from build123d import *

# Parameters (mm, degrees)
SKETCH1_R                = 1.75
SKETCH1_W                = 7.2
SKETCH1_H                = 5.4
BOSS_EXTRUDE1_DEPTH      = 5
FILLET5_RADIUS           = 10
FILLET5_LENGTH           = 5
FILLET2_R                = 5.4
FILLET6_R                = 5.4
SKETCH3_W                = 35
SKETCH3_H                = 20
SKETCH3_W_2              = 23
SKETCH3_H_2              = 13
BOSS_EXTRUDE4_DEPTH      = 5
SKETCH5_W                = 23
SKETCH5_H                = 13
CUT_EXTRUDE1_DEPTH       = 2.74
CUT_EXTRUDE2_DEPTH       = 76.166481892
FILLET9_R                = 4
BOSS_EXTRUDE7_DEPTH      = 26
BOSS_EXTRUDE7_DEPTH_BACK = 5
SKETCH7_W                = 5
SKETCH7_H                = 20
SKETCH8_R                = 2.75
CUT_EXTRUDE3_DEPTH       = 79.677569866
FILLET10_R               = 10
SKETCH9_R                = 1
CUT_EXTRUDE4_DEPTH       = 7
BOSS_EXTRUDE8_DEPTH      = 5
SKETCH11_R               = 1.3
CUT_EXTRUDE5_DEPTH       = 5
SKETCH12_W               = 14
SKETCH12_H               = 7
CUT_EXTRUDE6_DEPTH       = 4
FILLET11_R               = 3.5


with BuildPart() as part:
    # Sketch1 → Boss-Extrude1 (new body)
    # profile 1 of 4: a face of its own
    with BuildSketch(Plane(origin=(0, 0, 0), x_dir=(1, 0, 0), z_dir=(0, 1, 0))):
        with BuildLine():
            Line((3.05, 25), (0, 25))
            Line((0, 25), (0, 15))
            Line((0, 15), (10, 0))
            Line((10, 0), (26, 0))
            Line((26, 0), (36, 15))
            Line((36, 15), (60, 15))
            Line((60, 15), (60, 25))
            Line((60, 25), (44.5, 25))
            Line((44.5, 25), (44.5, 19.6))
            Line((44.5, 19.6), (37.3, 19.6))
            Line((37.3, 19.6), (26.5, 19.6))
            Line((26.5, 19.6), (26.5, 25))
            Line((26.5, 25), (6.55, 25))
            ThreePointArc((6.55, 25), (4.8, 23.25), (3.05, 25))
        make_face()
        with Locations(Location((13, 5, 0), (0, 0, 270))):
            Circle(SKETCH1_R, mode=Mode.SUBTRACT)
        with Locations(Location((23, 5, 0), (0, 0, 270))):
            Circle(SKETCH1_R, mode=Mode.SUBTRACT)
    # profile 2 of 4: a face of its own
    with BuildSketch(Plane(origin=(0, 0, 0), x_dir=(1, 0, 0), z_dir=(0, 1, 0))):
        with BuildLine():
            Line((10, 45), (0, 33.819660113))
            Line((0, 33.819660113), (0, 25))
            Line((0, 25), (3.05, 25))
            ThreePointArc((3.05, 25), (4.8, 26.75), (6.55, 25))
            Line((6.55, 25), (26.5, 25))
            Line((26.5, 25), (26.5, 30.4))
            Line((26.5, 30.4), (37.3, 30.4))
            Line((37.3, 30.4), (44.5, 30.4))
            Line((44.5, 30.4), (44.5, 25))
            Line((44.5, 25), (60, 25))
            Line((60, 25), (60, 35))
            Line((60, 35), (36, 35))
            Line((36, 35), (26, 45))
            Line((26, 45), (10, 45))
        make_face()
    # profile 3 of 4: a face of its own
    with BuildSketch(Plane(origin=(0, 0, 0), x_dir=(1, 0, 0), z_dir=(0, 1, 0))):
        with Locations((40.9, 27.7)):
            Rectangle(SKETCH1_W, SKETCH1_H)
    # profile 4 of 4: a face of its own
    with BuildSketch(Plane(origin=(0, 0, 0), x_dir=(1, 0, 0), z_dir=(0, 1, 0))):
        with Locations((40.9, 22.3)):
            Rectangle(SKETCH1_W, SKETCH1_H)
    extrude(amount=BOSS_EXTRUDE1_DEPTH)

    # Fillet5: full round fillet: the end face becomes a half cylinder, R = half its width
    fillet5_face = Plane((60, 2.5, -25), x_dir=(0, -1, 0), z_dir=(1, 0, 0))  # on the end face: x along it, z out of the body
    fillet5_slab = fillet5_face.offset(-FILLET5_RADIUS / 2) * Box(FILLET5_LENGTH, 2 * FILLET5_RADIUS, FILLET5_RADIUS, mode=Mode.PRIVATE)  # the body's end, R deep
    fillet5_round = Plane((50, 2.5, -25), x_dir=(1, 0, 0), z_dir=(0, -1, 0)) * Cylinder(FILLET5_RADIUS, FILLET5_LENGTH, mode=Mode.PRIVATE)  # its axis R under the face
    add(fillet5_slab - fillet5_round, mode=Mode.SUBTRACT)

    # Fillet2
    fillet2_edges = [part.edges().sort_by_distance(p)[0] for p in [
        (26.5, 2.5, -30.4),
        (26.5, 2.5, -19.6),
    ]]
    fillet(fillet2_edges, radius=FILLET2_R - 0.0001)  # a hair under: the kernel refuses the full size

    # Fillet6
    fillet6_edges = [part.edges().sort_by_distance(p)[0] for p in [
        (37.3, 2.5, -19.6),
        (37.3, 2.5, -30.4),
    ]]
    fillet(fillet6_edges, radius=FILLET6_R - 0.0001)  # a hair under: the kernel refuses the full size

    # Sketch3 → Boss-Extrude4 (add)
    with BuildSketch(Plane.XZ):
        with Locations((26.9, -25)):
            Rectangle(SKETCH3_W, SKETCH3_H)
        with Locations((26.9, -25)):
            Rectangle(SKETCH3_W_2, SKETCH3_H_2, mode=Mode.SUBTRACT)
    extrude(amount=BOSS_EXTRUDE4_DEPTH)

    # Sketch5 → Cut-Extrude1 (cut)
    with BuildSketch(Plane.XZ):
        with Locations((26.9, -25)):
            Rectangle(SKETCH5_W, SKETCH5_H)
    extrude(amount=-CUT_EXTRUDE1_DEPTH, mode=Mode.SUBTRACT)

    # Sketch6 → Cut-Extrude2 (cut, through all)
    with BuildSketch(Plane.XZ):
        with BuildLine():
            Line((44.4, -35), (50, -35))
            ThreePointArc((50, -35), (60, -25), (50, -15))
            Line((50, -15), (44.4, -15))
            Line((44.4, -15), (44.4, -35))
        make_face()
    extrude(amount=-CUT_EXTRUDE2_DEPTH, mode=Mode.SUBTRACT)

    # Fillet9
    fillet9_edges = [part.edges().sort_by_distance(p)[0] for p in [
        (44.4, 0, -35),
        (44.4, 0, -15),
    ]]
    fillet(fillet9_edges, radius=FILLET9_R)

    # Sketch7 → Boss-Extrude7 (add, two sides: drawn at the far end of the back side and taken through both)
    with BuildSketch(Plane(origin=(0, 0, -45), x_dir=(-1, 0, 0), z_dir=(0, 0, -1)).offset(-BOSS_EXTRUDE7_DEPTH_BACK)):
        with Locations((-11.5, -5)):
            Rectangle(SKETCH7_W, SKETCH7_H)
    extrude(amount=BOSS_EXTRUDE7_DEPTH + BOSS_EXTRUDE7_DEPTH_BACK)

    # Sketch8 → Cut-Extrude3 (cut, through all)
    with BuildSketch(Plane(origin=(14, 0, 0), x_dir=(0, 0, -1), z_dir=(1, 0, 0))):
        with Locations(Location((55.5, -4, 0), (0, 0, 90))):
            Circle(SKETCH8_R)
    extrude(amount=-CUT_EXTRUDE3_DEPTH, mode=Mode.SUBTRACT)

    # Fillet10
    fillet10_edges = [part.edges().sort_by_distance(p)[0] for p in [
        (11.5, -15, -71),
        (11.5, 5, -71),
    ]]
    fillet(fillet10_edges, radius=FILLET10_R - 0.0001)  # a hair under: the kernel refuses the full size

    # Sketch9 → Cut-Extrude4 (cut)
    with BuildSketch(Plane.XZ.offset(5)):
        with Locations(Location((13.1, -25, 0), (0, 0, 270))):
            Circle(SKETCH9_R)
        with Locations(Location((40.7, -25, 0), (0, 0, 270))):
            Circle(SKETCH9_R)
    extrude(amount=-CUT_EXTRUDE4_DEPTH, mode=Mode.SUBTRACT)

    # Sketch10 → Boss-Extrude8 (add)
    with BuildSketch(Plane.ZY.offset(-9)):
        Polygon((-40, 0), (-40, -15), (-35, -5), (-35, 0), align=None)
    extrude(amount=-BOSS_EXTRUDE8_DEPTH)

    # Sketch11 → Cut-Extrude5 (cut)
    with BuildSketch(Plane.ZY.offset(-9)):
        with Locations(Location((-51, -4, 0), (0, 0, 270))):
            Circle(SKETCH11_R)
        with Locations(Location((-60, -4, 0), (0, 0, 270))):
            Circle(SKETCH11_R)
    extrude(amount=-CUT_EXTRUDE5_DEPTH, mode=Mode.SUBTRACT)

    # Sketch12 → Cut-Extrude6 (cut)
    with BuildSketch(Plane.ZY.offset(-9)):
        with Locations((-55.6871773, -4.003401726)):
            Rectangle(SKETCH12_W, SKETCH12_H)
    extrude(amount=-CUT_EXTRUDE6_DEPTH, mode=Mode.SUBTRACT)

    # Fillet11
    fillet11_edges = [part.edges().sort_by_distance(p)[0] for p in [
        (11, -7.503401726, -48.6871773),
        (11, -0.503401726, -48.6871773),
        (11, -0.503401726, -62.6871773),
        (11, -7.503401726, -62.6871773),
    ]]
    fillet(fillet11_edges, radius=FILLET11_R - 0.0001)  # a hair under: the kernel refuses the full size


solid = part.part
Work out the finished part from the listing and answer in its coordinate system (mm). A direction names the side the tool comes from. Round coordinates to 2 decimals unless told otherwise and drop trailing zeros. Write each loop counter-clockwise with the first axis right and the second up, starting at its lowest first coordinate (ties: lowest second). Pieces come first, ordered by that corner, then holes. Notation, with made-up numbers: (0.5, 61.5) - (10.5, 61.5) arc R27 ccw to (10.5, 91.5) - close; hole circle Ø9 at (-6, 64.5). An arc over 180 degrees is marked (long way). Answer in a Markdown table with one row per item. Add a question column.
1. A cutting plane is placed at B-B, the plane y = 1. Determine the outline of the cut face in (x, z), and give its area (3 significant figures).
2. A cutting plane is placed at A-A, the plane x = 4. Determine the outline of the cut face in (y, z).
3. Given pin 1 (22 mm diameter, centred on x = 30.5, z = -28.5, fed in from -Y); pin 2 (2.5 mm diameter, centred on x = 31, y = -1.5, fed in from -Z); pin 3 (8 mm diameter, centred on x = 37, y = 1.5, fed in from -Z), each flat-ended and moving along its own axis, determine where each tip first touches the part or whether it passes through.
4. The mould has two halves that part along Z. Classify faces 1 (the flat face through (11.465, -10.07, -37.535)), 2 (the flat face through (27, -5, -32)), 3 (the flat face through (11, -0.503, -56)): +Z half, -Z half, draft (parallel to the pull), parting line (faces both ways), or undercut.
5. Find the intervals of material crossed by line 1 along X through (y, z) = (3.15, -25); line 2 along X through (y, z) = (-2.5, -25); line 3 along X through (y, z) = (0.25, -29.5), in increasing order. Write a range as from..to.
6. A cutting plane is placed at C-C, the plane z = -8.5. Determine the outline of the cut face in (x, y), and give its area (3 significant figures).
7. For faces 4 (the cylindrical face through (28.04, 3.886, -28.776)), 5 (the flat face through (27, -1, -31.5)), 6 (the cylindrical face through (11.028, -6.505, -49.74)), 7 (the flat face through (25, -2, -15)), 8 (the flat face through (22, 0, -40)), determine the directions among +Z, -Z, +X, -X, +Y, -Y from which every point of the face is accessible in a straight line to the end or side of a thin tool.
8. A cutting plane is placed at D-D, the plane y = -13.5. Determine the outline of the cut face in (x, z), and give its area (3 significant figures).
Worked out:
| question | item | result |
|---|---|---|
| 1 | outline | (0, -33.82) - (9, -43.88) - (9, -69) - (14, -69) - (14, -45) - (26, -45) - (36, -35) - (40.4, -35) arc R4 ccw to (44.4, -31) - (44.4, -19) arc R4 ccw to (40.4, -15) - (36, -15) - (26, 0) - (10, 0) - (0, -15) - close; hole circle Ø3.5 at (4.8, -25); hole circle Ø3.5 at (13, -5); hole circle Ø2 at (13.1, -25); hole (15.4, -31.5) - (38.4, -31.5) - (38.4, -18.5) - (15.4, -18.5) - close; hole circle Ø3.5 at (23, -5); hole circle Ø2 at (40.7, -25) |
| 1 | area | 1,310 mm^2 |
| 2 | outline | (0, -38.29) - (5, -38.29) - (5, -26.56) - (0, -26.56) - close; (0, -23.44) - (5, -23.44) - (5, -9) - (0, -9) - close |
| 3 | pin 1 | y = -5 |
| 3 | pin 2 | z = -35 |
| 3 | pin 3 | z = -38 |
| 4 | face 1 | +Z half |
| 4 | face 2 | draft |
| 4 | face 3 | undercut |
| 5 | line 1 | 0..3.05, 6.55..26.5, 37.3..44.4 |
| 5 | line 2 | 9.4..12.1, 14.1..15.4, 38.4..39.7, 41.7..44.4 |
| 5 | line 3 | 0..15.4, 38.4..44.4 |
| 6 | outline | (4.33, 0) - (31.67, 0) - (31.67, 5) - (4.33, 5) - close |
| 6 | area | 137 mm^2 |
| 7 | face 4 | +Y, -Y |
| 7 | face 5 | -Y |
| 7 | face 6 | -X |
| 7 | face 7 | +Z, +X, -Y |
| 7 | face 8 | -Z, +X, -Y |
| 8 | outline | (9, -66.27) - (14, -66.27) - (14, -39.25) - (9, -39.25) - close |
| 8 | area | 135 mm^2 |
